from build123d import *

# Parameters (mm, degrees)
F0_W      = 2.11328
F0_H      = 17.78
F1_DEPTH  = 1.5875
F3_DEPTH  = 5.588
F4_W      = 14.732
F4_H      = 38.1
F5_DEPTH  = 5.588
F3_FACE_W = 5.588
F3_FACE_H = 3.302
F6_DEPTH  = 0.508
F8_DEPTH  = 38.101
F9_W      = 5.08
F9_H      = 17.78
F10_DEPTH = 5.588
F12_DEPTH = 5.08
F14_DEPTH = 14.32052
F15_W     = 2.96672
F15_H     = 4.064
F16_DEPTH = 3.81
F17_W     = 5.3975
F17_H     = 4.064
F18_DEPTH = 2.11328
F20_DEPTH = 5.08


with BuildPart() as f1:
    # F0 (on Right) → F1 (new body)
    with BuildSketch(Plane.YZ):
        Polygon((11.43, 38.1), (-15.24, 38.1), (-15.24, 0), (11.43, 0), (11.43, 20.32), align=None)
        with Locations((12.48664, 29.21)):
            Rectangle(F0_W, F0_H)
    extrude(amount=F1_DEPTH)

    # F2 (on face) → F3 (join)
    with BuildSketch(Plane.YZ.offset(1.5875)):
        Polygon((3.556, 34.29), (0, 31.496), (0, 28.194), (3.556, 25.4), align=None)
        Polygon((3.556, 12.7), (0, 9.906), (0, 6.604), (3.556, 3.81), align=None)
    extrude(amount=F3_DEPTH)

    # F4 (on face) → F5 (join, through all)
    with BuildSketch(Plane.YZ.offset(1.5875)):
        with Locations((-7.874, 19.05)):
            Rectangle(F4_W, F4_H)
    extrude(amount=F5_DEPTH)

    # F3_face (on face) → F6 (join)
    with BuildSketch(Plane(origin=(4.3815, 0, 29.845), x_dir=(1, 0, 0), z_dir=(0, -1, 0))):
        Rectangle(F3_FACE_W, F3_FACE_H)
        with Locations((0, -21.59)):
            Rectangle(F3_FACE_W, F3_FACE_H)
    extrude(amount=F6_DEPTH)

    # F7 (on face) → F8 (cut, through all)
    with BuildSketch(Plane.XY.offset(38.1)):
        Polygon((3.81, -12.7), (3.81, -2.794), (0, -5.207), (0, -10.287), align=None)
    extrude(amount=-F8_DEPTH, mode=Mode.SUBTRACT)

    # F9 (on face) → F10 (join, through all)
    with BuildSketch(Plane.YZ.offset(1.5875)):
        with Locations((11.00328, 29.21)):
            Rectangle(F9_W, F9_H)
    extrude(amount=F10_DEPTH)

    # F11 (on face) → F12 (cut, through all)
    with BuildSketch(Plane(origin=(0, 13.54328, 0), x_dir=(-1, 0, 0), z_dir=(0, 1, 0))):
        Polygon((-7.1755, 28.194), (-7.1755, 20.32), (-1.0795, 20.32), align=None)
    extrude(amount=-F12_DEPTH, mode=Mode.SUBTRACT)

    # F13 (on face) → F14 (join)
    with BuildSketch(Plane(origin=(0, 13.54328, 0), x_dir=(-1, 0, 0), z_dir=(0, 1, 0))):
        Polygon((-3.6195, 36.068), (-7.1755, 33.274), (-7.1755, 29.972), (-3.6195, 27.178), align=None)
    extrude(amount=F14_DEPTH)

    # F15 (on face) → F16 (join)
    with BuildSketch(Plane.YZ.offset(1.5875)):
        with Locations((9.94664, 2.032)):
            Rectangle(F15_W, F15_H)
    extrude(amount=F16_DEPTH)

    # F17 (on face) → F18 (join, through all)
    with BuildSketch(Plane(origin=(0, 11.43, 0), x_dir=(-1, 0, 0), z_dir=(0, 1, 0))):
        with Locations((-2.69875, 2.032)):
            Rectangle(F17_W, F17_H)
    extrude(amount=F18_DEPTH)

    # F19 (on face) → F20 (cut, through all)
    with BuildSketch(Plane(origin=(0, 13.54328, 0), x_dir=(-1, 0, 0), z_dir=(0, 1, 0))):
        Polygon((-1.5875, 4.064), (-5.3975, 4.064), (-5.3975, 0), align=None)
    extrude(amount=-F20_DEPTH, mode=Mode.SUBTRACT)


solid = f1.part
Geometry check sheet. Reference: the model listing, model coordinates, mm. A direction names the side the tool comes from. Round coordinates to 2 decimals unless told otherwise and drop trailing zeros. Order: outer loops, then holes, each group sorted by start corner. A loop starts at its lowest first (then second) coordinate and runs counter-clockwise, first axis right, second up. Notation, with made-up numbers: (24.5, -26.75) -> (74.5, -26.75) arc R28 ccw to (74.5, 6.25) -> close; hole circle Ø4 at (67, 13). An arc over 180 degrees is marked (long way). Use one line per item in the form item = value.
1. Set-up check for faces 1 (the face through (4.34, 1.8, 32.91)), 2 (the face through (4.34, 1.75, 5.23)), 3 (the face through (5.422, 20.603, 28.595)): record each of +Z, -Z, +X, -X, +Y, -Y from which the full face is reachable in a straight line by a thin tool's end or side.
Working result:
face_1 = +Z, +X
face_2 = -Z, +X
face_3 = -Z, +X, +Y
2. Scan lines: line 1 along Y through (x, z) = (4, 24.5); line 2 along Y through (x, z) = (5, 30.5); line 3 along X through (y, z) = (4, 25.5). Record each from-to range of solid material in increasing order. Write a range as from..to.
Working result:
line_1 = -15.24..-0.51, 8.46..13.54
line_2 = -15.24..3.56, 8.46..27.86
line_3 = 0..1.59
3. Go/stop test with flat-tipped pins: pin 1 (1 mm diameter, centred on x = 2, y = 20, fed in from -Z); pin 2 (3.5 mm diameter, centred on y = 3, z = 21.5, fed in from +X); pin 3 (1.5 mm diameter, centred on x = 1.5, z = 26, fed in from +Y); pin 4 (2.5 mm diameter, centred on y = 19.5, z = 32.5, fed in from -X). Record where each tip stops, or that it passes through.
Working result:
pin_1 = through
pin_2 = 1.59
pin_3 = 13.54
pin_4 = 3.62
4. Mould release check, pull along Z, two halves, no side actions. Record for faces 4 (the face through (4, -1, 0)), 5 (the face through (3, 8.463, 2)), 6 (the face through (4.085, 11.039, 24.202)): pulls with the +Z half, pulls with the -Z half, needs draft (parallel to the pull), parting line crosses it, or undercut.
Working result:
face_4 = pulls with the -Z half
face_5 = needs draft
face_6 = undercut
5. Cross-section at A-A, the plane z = 9. Enter the section's corners in (x, y), plus the area to 3 significant figures.
Working result:
outline = (0, -15.24) -> (7.18, -15.24) -> (7.18, 3.56) -> (1.59, 3.56) -> (1.59, 11.43) -> (0, 11.43) -> (0, -5.21) -> (3.81, -2.79) -> (3.81, -12.7) -> (0, -10.29) -> close
area = 119 mm^2
6. Cross-section at D-D, the plane y = 19.5. Enter the section's corners in (x, z).
Working result:
outline = (3.62, 27.18) -> (7.18, 29.97) -> (7.18, 33.27) -> (3.62, 36.07) -> close
7. Cross-section at B-B, the plane x = 0.5. Enter the section's corners in (y, z), plus the area to 3 significant figures.
Working result:
outline = (-15.24, 0) -> (-10.6, 0) -> (-10.6, 38.1) -> (-15.24, 38.1) -> close; (-4.89, 0) -> (13.54, 0) -> (13.54, 4.06) -> (11.43, 4.06) -> (11.43, 20.32) -> (13.54, 20.32) -> (13.54, 38.1) -> (-4.89, 38.1) -> close
area = 845 mm^2
8. Cross-section at C-C, the plane x = 4.75. Enter the section's corners in (y, z).
Working result:
outline = (-15.24, 0) -> (-0.51, 0) -> (-0.51, 6.6) -> (0, 6.6) -> (3.56, 3.81) -> (3.56, 12.7) -> (0, 9.91) -> (-0.51, 9.91) -> (-0.51, 28.19) -> (0, 28.19) -> (3.56, 25.4) -> (3.56, 34.29) -> (0, 31.5) -> (-0.51, 31.5) -> (-0.51, 38.1) -> (-15.24, 38.1) -> close; (8.46, 0) -> (13.54, 0) -> (13.54, 0.69) -> (8.46, 0.69) -> close; (8.46, 25.06) -> (13.54, 25.06) -> (13.54, 28.07) -> (27.86, 28.07) -> (27.86, 35.18) -> (13.54, 35.18) -> (13.54, 38.1) -> (8.46, 38.1) -> close
